```python
from build123d import *

# Parameters (mm, degrees)
SKETCH1_R               = 1.5
SKETCH1_W               = 5
SKETCH1_H               = 2
BOSS_EXTRUDE1_DEPTH     = 5
SENSOR_POS_R            = 1.5
SENSOR_POS_W            = 2.5
SENSOR_POS_H            = 10
SENSOR_POS_W_2          = 19
SENSOR_POS_H_2          = 4
SENSOR_POS_W_3          = 10
SENSOR_POS_H_3          = 2.5
CUT_EXTRUDE1_DEPTH      = 220.265652723
CUT_EXTRUDE2_DEPTH      = 220.265652723
CUT_EXTRUDE2_DEPTH_BACK = 220.265652723
SKETCH2_R               = 1.5


with BuildPart() as part:
    # Sketch1 → Boss-Extrude1 (new body)
    with BuildSketch(Plane(origin=(0, 0, 0), x_dir=(1, 0, 0), z_dir=(0, 1, 0))):
        Polygon((55, -190.411113167), (64, -181.411113167), (64, -161.411113167), (54, -170.577779834), (54, -176.577779834), (41, -184.083333333), (37.5, -184.083333333), (35, -181.583333333), (35, -131.583333333), (40, -127), (52, -127), (64, -116), (64, -66), (70, -60), (70, -40), (65, -40), (65, -30), (70, -30), (70, 0), (-70, 0), (-70, -30), (-65, -30), (-65, -40), (-70, -40), (-70, -60), (-64, -66), (-64, -116), (-52, -127), (-40, -127), (-35, -131.583333333), (-35, -181.583333333), (-37.5, -184.083333333), (-41, -184.083333333), (-54, -176.577779834), (-54, -170.577779834), (-64, -161.411113167), (-64, -181.411113167), (-55, -190.411113167), (-25, -207.731621243), (25, -207.731621243), align=None)
        with Locations(Location((59, -5, 0), (0, 0, 270))):
            Circle(SKETCH1_R, mode=Mode.SUBTRACT)
        with Locations(Location((59, -71, 0), (0, 0, 270))):
            Circle(SKETCH1_R, mode=Mode.SUBTRACT)
        with Locations(Location((59, -111, 0), (0, 0, 270))):
            Circle(SKETCH1_R, mode=Mode.SUBTRACT)
        with Locations(Location((-59, -111, 0), (0, 0, 90))):
            Circle(SKETCH1_R, mode=Mode.SUBTRACT)
        with Locations(Location((-59, -71, 0), (0, 0, 90))):
            Circle(SKETCH1_R, mode=Mode.SUBTRACT)
        with Locations(Location((-59, -5, 0), (0, 0, 90))):
            Circle(SKETCH1_R, mode=Mode.SUBTRACT)
        with Locations((52.5, -21.5)):
            Rectangle(SKETCH1_W, SKETCH1_H, mode=Mode.SUBTRACT)
        with Locations((40, -21.5)):
            Rectangle(SKETCH1_W, SKETCH1_H, mode=Mode.SUBTRACT)
        with Locations((27.5, -21.5)):
            Rectangle(SKETCH1_W, SKETCH1_H, mode=Mode.SUBTRACT)
        with Locations((52.5, -48.5)):
            Rectangle(SKETCH1_W, SKETCH1_H, mode=Mode.SUBTRACT)
        with Locations((40, -48.5)):
            Rectangle(SKETCH1_W, SKETCH1_H, mode=Mode.SUBTRACT)
        with Locations((27.5, -48.5)):
            Rectangle(SKETCH1_W, SKETCH1_H, mode=Mode.SUBTRACT)
        with Locations((-52.5, -48.5)):
            Rectangle(SKETCH1_W, SKETCH1_H, mode=Mode.SUBTRACT)
        with Locations((-40, -48.5)):
            Rectangle(SKETCH1_W, SKETCH1_H, mode=Mode.SUBTRACT)
        with Locations((-27.5, -48.5)):
            Rectangle(SKETCH1_W, SKETCH1_H, mode=Mode.SUBTRACT)
        with Locations((-52.5, -21.5)):
            Rectangle(SKETCH1_W, SKETCH1_H, mode=Mode.SUBTRACT)
        with Locations((-40, -21.5)):
            Rectangle(SKETCH1_W, SKETCH1_H, mode=Mode.SUBTRACT)
        with Locations((-27.5, -21.5)):
            Rectangle(SKETCH1_W, SKETCH1_H, mode=Mode.SUBTRACT)
    extrude(amount=BOSS_EXTRUDE1_DEPTH)

    # Sensor Pos → Cut-Extrude1 (cut, through all)
    with BuildSketch(Plane.XZ):
        with Locations(Location((27.5, 153.231621243, 0), (0, 0, 270))):
            Circle(SENSOR_POS_R)
        with Locations(Location((-27.5, 153.231621243, 0), (0, 0, 270))):
            Circle(SENSOR_POS_R)
        with Locations(Location((-21, 190.731621243, 0), (0, 0, 270))):
            Circle(SENSOR_POS_R)
        with Locations(Location((21, 190.731621243, 0), (0, 0, 270))):
            Circle(SENSOR_POS_R)
        with Locations((-33.75, 153.731621243)):
            Rectangle(SENSOR_POS_W, SENSOR_POS_H)
        with Locations((33.75, 153.731621243)):
            Rectangle(SENSOR_POS_W, SENSOR_POS_H)
        with Locations((18.7, 129.291666667)):
            Rectangle(SENSOR_POS_W_2, SENSOR_POS_H_2)
        with Locations((-11.666666667, 171.231621243)):
            Rectangle(SENSOR_POS_W_3, SENSOR_POS_H_3)
        with Locations((11.666666667, 171.231621243)):
            Rectangle(SENSOR_POS_W_3, SENSOR_POS_H_3)
    extrude(amount=-CUT_EXTRUDE1_DEPTH, mode=Mode.SUBTRACT)

    # Sketch2 → Cut-Extrude2 (cut, two sides: drawn at the far end of the back side and taken through both)
    with BuildSketch(Plane(origin=(0, 5, 0), x_dir=(1, 0, 0), z_dir=(0, 1, 0)).offset(-CUT_EXTRUDE2_DEPTH_BACK)):
        with Locations(Location((-51, -63, 0), (0, 0, 270))):
            Circle(SKETCH2_R)
        with Locations(Location((-14, -63, 0), (0, 0, 270))):
            Circle(SKETCH2_R)
        with Locations(Location((-51, -100, 0), (0, 0, 270))):
            Circle(SKETCH2_R)
        with Locations(Location((-14, -100, 0), (0, 0, 270))):
            Circle(SKETCH2_R)
        with Locations(Location((51, -56, 0), (0, 0, 270))):
            Circle(SKETCH2_R)
        with Locations(Location((-3, -120, 0), (0, 0, 270))):
            Circle(SKETCH2_R)
        with Locations(Location((51, -120, 0), (0, 0, 270))):
            Circle(SKETCH2_R)
    extrude(amount=CUT_EXTRUDE2_DEPTH + CUT_EXTRUDE2_DEPTH_BACK, mode=Mode.SUBTRACT)


solid = part.part
```
Source: CAD feature listing. Evaluate the final solid. Frame: model axes, mm. A direction names the side the tool comes from. Round coordinates to 2 decimals unless told otherwise and drop trailing zeros. Loops run counter-clockwise (first coordinate to the right, second up) from the corner with the lowest first, then second, coordinate; pieces in that order, holes last.
(1) Section query A-A (z = 167). Output: boundary loops of the cut face in (x, y), and give its area (3 significant figures).
From the geometry:
outline: (-64, 0) - (-57.9, 0) - (-57.9, 5) - (-64, 5) - close; (-35, 0) - (35, 0) - (35, 5) - (-35, 5) - close; (57.9, 0) - (64, 0) - (64, 5) - (57.9, 5) - close
area: 411 mm2
(2) Access query for faces 1 (the flat face through (40, 2, 47.5)), 2 (the flat face through (-64, 2, 91)), 3 (the flat face through (67, 2, 30)). Directions: +Z, -Z, +X, -X, +Y, -Y. A direction counts if a zero-diameter tool reaches every point of the face in a straight line with its end or side. Return the directions, or none.
From the geometry:
face 1: +Y, -Y
face 2: +Z, -X, +Y, -Y
face 3: +X, +Y, -Y
(3) Material intervals for probe 1 along Z at (x, y) = (16.5, 1.5); probe 2 along X at (y, z) = (1.8, 111); probe 3 along X at (y, z) = (3.6, 5), sorted ascending.
From the geometry:
probe 1: z = 0 to 127.29, 131.29 to 169.98, 172.48 to 207.73
probe 2: x = -64 to -60.5, -57.5 to 57.5, 60.5 to 64
probe 3: x = -70 to -60.5, -57.5 to 57.5, 60.5 to 70
(4) Pull-direction query (Z, two-part tool) for faces 4 (the flat face through (27, 2, 22.5)), 5 (the flat face through (-1, 0, 79)), 6 (the flat face through (-40.21, 2.46, 198.95)); classes: +Z half, -Z half, draft (parallel to the pull), parting line (faces both ways), or undercut.
From the geometry:
face 4: undercut
face 5: draft
face 6: +Z half
(5) Contact query for flat-ended pins moving along their axis: pin 1 Ø1.5 at (x, y) = (41, 2.5) entering from +Z; pin 2 Ø1.5 at (y, z) = (3.5, 113.5) entering from -X; pin 3 Ø1.8 at (x, z) = (-51, 100) entering from +Y; pin 4 Ø1 at (y, z) = (1, 120.5) entering from -X. Output: stop coordinate, or through.
From the geometry:
pin 1: stops at z = 198.93
pin 2: stops at x = -64
pin 3: passes through
pin 4: stops at x = -59.64
(6) Section query B-B (y = 1.05). Give the number of separate pieces and of enclosed holes in the cut face, and give its area (3 significant figures).
From the geometry:
separate pieces: 1
enclosed holes: 32
area: 23,000 mm2
